from build123d import *

# Parameters (mm, degrees)
BOSS_EXTRUDE1_DEPTH = 1.5
SKETCH2_R           = 5
CUT_EXTRUDE1_DEPTH  = 142.810613143


with BuildPart() as part:
    # Sketch1 → Boss-Extrude1 (new, symmetric)
    with BuildSketch(Plane(origin=(0, 0, 0), x_dir=(0, 0, -1), z_dir=(1, 0, 0))):
        with BuildLine():
            ThreePointArc((0, 79), (11, 90), (0, 101))
            ThreePointArc((0, 101), (-25.350874614, 97.701945149), (-49.014054674, 88.027343403))
            ThreePointArc((-49.014054674, 88.027343403), (-68.978437503, 67.692387852), (-75.252234106, 39.89442974))
            ThreePointArc((-75.252234106, 39.89442974), (-79.876334442, -1.725579257), (-97.797422275, -39.573195612))
            ThreePointArc((-97.797422275, -39.573195612), (-94.917356951, -53.128320897), (-81.574017035, -49.387802533))
            ThreePointArc((-81.574017035, -49.387802533), (-66.010073659, -10.395208993), (-58.530464131, 30.917187762))
            ThreePointArc((-58.530464131, 30.917187762), (-46.946256543, 59.483246729), (-21.037120215, 76.184451628))
            ThreePointArc((-21.037120215, 76.184451628), (-10.612348227, 78.292988751), (0, 79))
        make_face()
    extrude(amount=BOSS_EXTRUDE1_DEPTH, both=True)

    # Sketch2 → Cut-Extrude1 (cut, through all)
    with BuildSketch(Plane(origin=(1.5, 0, 0), x_dir=(0, 0, -1), z_dir=(1, 0, 0))):
        with Locations((0, 90)):
            Circle(SKETCH2_R)
        with Locations((-90, -45)):
            Circle(SKETCH2_R)
    extrude(amount=-CUT_EXTRUDE1_DEPTH, mode=Mode.SUBTRACT)


solid = part.part
Design review of the part built by this model. Coordinates are the model's own, in mm. Give positions to 0.01 mm unless a question says otherwise; leave off trailing zeros. Loops run counter-clockwise (first coordinate to the right, second up) from the corner with the lowest first, then second, coordinate; pieces in that order, holes last. Notation, with made-up numbers: M 26,76.5 L 35,76.5 A32 ccw 35,109.5 Z; hole C -17.75,63.25 d5. An arc over 180 degrees is marked long. One line per question, with ' | ' between items. Start each with the question number.
1. Add section D-D (z = 10.5). Write out the cut boundary in (x, y), plus the area to 3 significant figures.
2. The part is to be moulded in two halves that separate along Y. For faces 1 (the face through (0, -41, 87)), 2 (the face through (0.021, 97.793, 25.004)), 3 (the face through (0.021, -53.014, 95.102)), 4 (the face through (0.021, -1.159, 79.717)), say which applies: released by +Y, released by -Y, zero draft, split by the parting line, or undercut.
3. Add section C-C (x = 0.5). Write out the cut boundary in (y, z), plus the area to 3 significant figures.
4. Add section A-A (y = 90). Write out the cut boundary in (x, z), plus the area to 3 significant figures.
5. Add section B-B (z = 90). Write out the cut boundary in (x, y), plus the area to 3 significant figures.
6. Insertion check: P1, Ø1, axis at x = 0.5, z = 19.5, coming from the +Y side; P2, Ø1.5, axis at x = 0.5, y = -2.5, coming from the +Z side; P3, Ø6, axis at y = 90, z = 0, coming from the -X side. Each pin has a flat end and moves straight along its axis. Give the tip position at first contact, or say it passes through.
7. To check wall thickness, follow L1, parallel to Y at x = 1.3, z = 90.5; L2, parallel to Y at x = 0.7, z = 90; L3, parallel to Z at x = 0.15, y = -19. State the ranges of each line that lie inside material, in increasing order.
Worked out:
1) outline: M -1.5,78.31 L 1.5,78.31 L 1.5,100.44 L -1.5,100.44 Z | area: 66.4 mm²
2) face 1: undercut | face 2: released by +Y | face 3: split by the parting line | face 4: undercut
3) outline: M -49.39,81.57 A209.58 ccw 30.92,58.53 A51.09 cw 76.18,21.04 A80 cw 79,0 A11 ccw 101,0 A99.08 ccw 88.03,49.01 A52.08 ccw 39.89,75.25 A126.87 cw -39.57,97.8 A9.5 ccw long Z; hole C -45,90 d10; hole C 90,0 d10 | area: 3,670 mm²
4) outline: M -1.5,-11 L 1.5,-11 L 1.5,-5 L -1.5,-5 Z; M -1.5,5 L 1.5,5 L 1.5,45.37 L -1.5,45.37 Z | area: 139 mm²
5) outline: M -1.5,-54.5 L 1.5,-54.5 L 1.5,-50 L -1.5,-50 Z; M -1.5,-40 L 1.5,-40 L 1.5,-26.83 L -1.5,-26.83 Z | area: 53.0 mm²
6) P1: stops at y = 99.16 | P2: stops at z = 80.32 | P3: passes through
7) L1: y = -54.49 to -49.97, -40.03 to -27.76 | L2: y = -54.5 to -50, -40 to -26.83 | L3: z = 68.68 to 86.16
